from build123d import *

# Parameters (mm, degrees)
F0_W     = 12.7625
F0_H     = 117.8206766
F0_R     = 4
F0_R_2   = 1.35255
F0_W_2   = 8
F0_H_2   = 79.9424962
F1_DEPTH = 6.35
F2_R     = 0.79375
F3_SIZE  = 0.254
F4_R     = 1.35255
F5_DEPTH = 8.0325436313


# Not quite as in the source:
# - a feature names something its author has since deleted; it is built from what else it names


with BuildPart() as f1:
    # F0 (on Top) → F1 (new body)
    with BuildSketch(Plane.XY):
        with Locations((0, -2.2078402)):
            Rectangle(F0_W, F0_H)
        with Locations((0, -50.3212481)):
            Circle(F0_R, mode=Mode.SUBTRACT)
        with Locations((0, -43.1462481)):
            Circle(F0_R_2, mode=Mode.SUBTRACT)
        Rectangle(F0_W_2, F0_H_2, mode=Mode.SUBTRACT)
        with Locations((0, 43.1462481)):
            Circle(F0_R_2, mode=Mode.SUBTRACT)
        with Locations((0, 50.3212481)):
            Circle(F0_R, mode=Mode.SUBTRACT)
    extrude(amount=F1_DEPTH)

    # F2
    f2_edges = [f1.edges().sort_by_distance(p)[0] for p in [
        (4, -39.971248, 3.175),
        (-4, -39.971248, 3.175),
        (-4, 39.971248, 3.175),
        (4, 39.971248, 3.175),
    ]]
    fillet(f2_edges, radius=F2_R)

    # F3
    f3_edges = [f1.edges().sort_by_distance(p)[0] for p in [
        (-4, 50.321248, 6.35),
        (-4, -50.321248, 6.35),
    ]]
    chamfer(f3_edges, length=F3_SIZE)

    # F4 (on face) → F5 (cut, up to face)
    with BuildSketch(Plane.XZ.offset(61.1181785)):
        with Locations((0, 3.175)):
            Circle(F4_R)
    extrude(amount=-F5_DEPTH, mode=Mode.SUBTRACT)


solid = f1.part
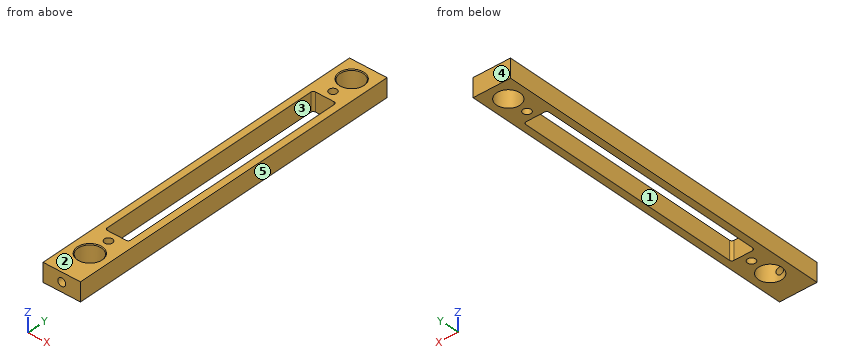
Source: CAD feature listing. Evaluate the final solid. Frame: model axes, mm. Face numbers are marked on the shaded views. A direction names the side the tool comes from. Give positions to 0.01 mm unless a question says otherwise; leave off trailing zeros. Order: outer loops, then holes, each group sorted by start corner. A loop starts at its lowest first (then second) coordinate and runs counter-clockwise, first axis right, second up. Notation, with made-up numbers: (84.5, 26.25) -> (104.5, 26.25) arc R12 cw to (104.5, 39.25) -> close; hole circle Ø9 at (-8.5, -9). An arc over 180 degrees is marked (long way). Write item = value, one per line.
Q1. Cut plane A-A, the plane y = -9. Output: boundary loops of the cut face in (x, z).
Data:
outline = (-6.38, 0) -> (-4, 0) -> (-4, 6.35) -> (-6.38, 6.35) -> close; (4, 0) -> (6.38, 0) -> (6.38, 6.35) -> (4, 6.35) -> close
Q2. Pull-direction query (Y, two-part tool) for the marked faces 3, 4 and 5; classes: released by +Y, released by -Y, zero draft, split by the parting line, or undercut.
Data:
face_3 = undercut
face_4 = released by +Y
face_5 = zero draft
Q3. Cut plane B-B, the plane x = 0. State how many separate pieces and enclosed holes the cut face has, and give its area (3 significant figures).
Data:
separate_pieces = 7
enclosed_holes = 0
area = 86.1 mm^2
Q4. Set-up query: the marked faces 1 and 2. Return all of +Z, -Z, +X, -X, +Y, -Y with unobstructed straight access to the full face (end or side cutting, diameter ignored); none if empty.
Data:
face_1 = +Z, -Z
face_2 = +Z, +X, -X, +Y, -Y
Q5. Material intervals for line 1 (Y direction, x = 0, z = 2.5); line 2 (Y direction, x = 0.25, z = 0.5); line 3 (X direction, y = 3, z = 5.5), sorted ascending. Write a range as from..to.
Data:
line_1 = -46.32..-44.5, -41.79..-39.97, 39.97..41.79, 44.5..46.32, 54.32..56.7
line_2 = -61.12..-54.31, -46.33..-44.48, -41.82..-39.97, 39.97..41.82, 44.48..46.33, 54.31..56.7
line_3 = -6.38..-4, 4..6.38
